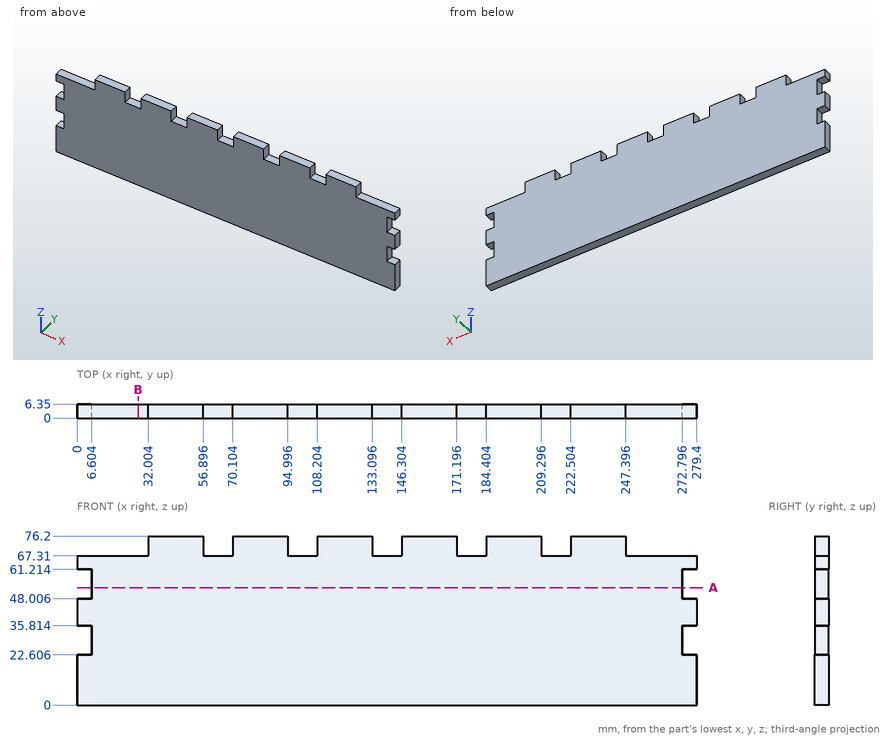
Source: three-view drawing plus pictorial views. Frame: mm from the lowest corner of the part. Round coordinates to 2 decimals unless told otherwise and drop trailing zeros. Order: outer loops, then holes, each group sorted by start corner. A loop starts at its lowest first (then second) coordinate and runs counter-clockwise, first axis right, second up. Notation, with made-up numbers: (-35.75, 26) -> (-25.75, 26) arc R28 ccw to (-25.75, 57) -> close; hole circle Ø2 at (1, -25.5). An arc over 180 degrees is marked (long way). Use CSV: the item, a comma, the result in double quotes. Start each with the question number.
1) Material intervals for line 1 along X through (y, z) = (1, 69.5); line 2 along Z through (x, y) = (173, 2.75); line 3 along X through (y, z) = (6, 30.5), sorted ascending. Write a range as from..to.
2) Section A-A (z = 53). Return the cut outline in (x, y).
3) First-contact query: pin 1 Ø1.9 at (x, y) = (258.5, 1.5) entering from +Z; pin 2 Ø1.9 at (y, z) = (4, 69.5) entering from +X; pin 3 Ø1 at (y, z) = (5, 49) entering from -X. Flat tips, straight axial feed; report the tip coordinate or a pass-through.
4) Section B-B (x = 27.5). Return the cut outline in (y, z), and give its area (3 significant figures).
Returned:
1,line 1,"x = 32..56.9, 70.1..95, 108.2..133.1, 146.3..171.2, 184.4..209.3, 222.5..247.4"
1,line 2,"z = 0..67.31"
1,line 3,"x = 6.6..272.8"
2,outline,"(6.6, 0) -> (272.8, 0) -> (272.8, 6.35) -> (6.6, 6.35) -> close"
3,pin 1,"stops at z = 67.31"
3,pin 2,"stops at x = 247.4"
3,pin 3,"stops at x = 6.6"
4,outline,"(0, 0) -> (6.35, 0) -> (6.35, 67.31) -> (0, 67.31) -> close"
4,area,"427 mm²"
